Can you work these out from the model? Positions are in its coordinate system, mm. A direction names the side the tool comes from. Round coordinates to 2 decimals unless told otherwise and drop trailing zeros. Order: outer loops, then holes, each group sorted by start corner. A loop starts at its lowest first (then second) coordinate and runs counter-clockwise, first axis right, second up.
Q1. For faces 4 (the face through (-0.6, 0.57, -48.48)), 5 (the face through (-47, 7, -23)), which set-ups out of +Z, -Z, +X, -X, +Y, -Y let a thin tool reach every point of the face, with its end or its side?
Q2. If we section it at A-A (y = 7.5): Count the separate pieces of the cut face and the enclosed holes in it, plus the area to 3 significant figures.
Q3. If I drill on line 1 (Y direction, x = -7, z = -49); line 2 (X direction, y = 7.5, z = -48.9) (3 decimals); line 3 (X direction, y = 7.5, z = -48.95), over which ranges is the centre line in solid material (lowest first)?
Q4. If we section it at B-B (z = -38): Please give me the cut outline in (x, y).
Q5. If we section it at C-C (x = -7): Please give me the cut outline in (y, z), plus the area to 3 significant figures.
Q6. Will this pin go through, and if not, where does the flat tip stop? P1, Ø1.5, axis at y = 8.5, z = -43.5, coming from the +X side.
Q7. If we section it at D-D (y = 11.5): Please give me the cut outline in (x, z).
Q8. We'd pull the mould along Y, two halves only. Please class faces 1 (the face through (-48, 7, 0)), 2 (the face through (-36.45, 6.69, -49.21)), 3 (the face through (-48.52, 14.4, -0.57)): pulls with the +Y half, pulls with the -Y half, needs draft (parallel to the pull), parting line crosses it, or undercut.
Autodesk Inventor part; units mm, degrees
ref_plane "YZ Plane" through (0, 0, 0) normal (1, 0, 0) x (0, 1, 0)
ref_plane "XZ Plane" through (0, 0, 0) normal (0, 1, 0) x (-1, 0, 0)
ref_plane "XY Plane" through (0, 0, 0) normal (0, 0, 1) x (1, 0, 0)
sketch "Sketch1" plane through (0, 0, 0) normal (0, 1, 0) x (-1, 0, 0)
  line L0 (0, 0) -> (50, 0)
  line L1 (50, 0) -> (50, -46)
  line L2 (46, -50) -> (0, -50)
  line L3 (0, -50) -> (0, 0)
  arc A0 (46, -50) -> (50, -46) centre (46, -46) ccw
  line L4 (0, 0) -> (47, 0)
  line L5 (47, 0) -> (47, -46)
  line L6 (46, -47) -> (0, -47)
  line L7 (0, -47) -> (0, 0)
  arc A1 (46, -47) -> (47, -46) centre (46, -46) ccw
  point P0 (50, -50)
  point P1 (47, -47)
  dimension "d0" = 50
  dimension "d1" = 50
  dimension "d2" = 4
  dimension "d3" = 47
  dimension "d4" = 47
  dimension "d5" = 1
extrude "Extrusion1" add sketch "Sketch1" along normal blind 15 contours L0 L1 A0 L2 L3 L6 A1 L5
fillet "Fillet1" radius 2 4 edges at (-48.5, 15, 0) (-48.5, 0, 0) (0, 15, -48.5) (0, 0, -48.5)
sketch "Sketch2" plane through (-47, 0, -46) normal (1, 0, 0) x (0, 0, -1)
  line L0 (-57.4618, 7.5) -> (28.1267, 7.5) construction
  line L1 (-46, 2) -> (-46, 13)
  point P0 (-46, 0)
  point P1 (-46, 7.5)
  point P2 (-39, 7.5)
  point P3 (-8, 7.5)
  dimension "d9" = 7
  dimension "d10" = 31
hole "Hole1" at (-47, 7.5, -7) at (-47, 7.5, -38) direction (-1, 0, 0) diameter 3.5 end through all countersink diameter 6.3 countersink angle 90
sketch "Sketch3" plane through (-46, 0, -47) normal (0, 0, 1) x (1, 0, 0)
  line L0 (63.5676, 7.5) -> (-29.6264, 7.5) construction
  line L1 (46, 2) -> (46, 13) construction
  arc A0 (44, 0) -> (46, 2) centre (44, 2) ccw
  line L2 (46, 2) -> (46, 13)
  arc A1 (46, 13) -> (44, 15) centre (44, 13) ccw
  line L3 (0, 15) -> (44, 15)
  line L4 (0, 0) -> (0, 15)
  line L5 (0, 0) -> (44, 0)
  point P0 (46, 0)
  point P1 (46, 7.5)
  point P2 (39, 7.5)
  point P3 (8, 7.5)
  dimension "d18" = 7
  dimension "d19" = 31
hole "Hole2" at (-7, 7.5, -47) at (-38, 7.5, -47) direction (0, 0, -1) diameter 3.5 end through all countersink diameter 6.3 countersink angle 90
properties part number "Right Bracket 50mm RS749-1680" material "Stainless Steel"
Solution:
1. face 4: +Z, -Z, +X, -Y
1. face 5: +Z, +X, +Y, -Y
2. separate pieces: 5
2. enclosed holes: 0
2. area: 238 mm2
3. line 1: y = 0 to 5.75, 9.25 to 15
3. line 2: x = -48.755 to -39.75, -36.25 to -8.75, -5.25 to 0
3. line 3: x = -48.7 to -39.75, -36.25 to -8.75, -5.25 to 0
4. outline: (-50, 0) - (-47, 0) - (-47, 4.35) - (-48.4, 5.75) - (-50, 5.75) - close; (-50, 9.25) - (-48.4, 9.25) - (-47, 10.65) - (-47, 15) - (-50, 15) - close
5. outline: (0, -50) - (5.75, -50) - (5.75, -48.4) - (4.35, -47) - (0, -47) - close; (9.25, -50) - (15, -50) - (15, -47) - (10.65, -47) - (9.25, -48.4) - close
5. area: 32.5 mm2
6. P1: stops at x = -47
7. outline: (-50, -46) arc R4 ccw to (-46, -50) - (0, -50) - (0, -47) - (-46, -47) arc R1 cw to (-47, -46) - (-47, 0) - (-50, 0) - close
8. face 1: needs draft
8. face 2: undercut
8. face 3: pulls with the +Y half
